from build123d import *

# Parameters (mm, degrees)
SKETCH_1_W          = 204
SKETCH_1_H          = 52
EXTRUDE_1_DEPTH     = 6
CUT_EXTRUDE_1_REACH = 107.432
SKETCH_2_R          = 1.6
SKETCH_2_R_2        = 4.5
FILLET_3_R          = 20


with BuildPart() as part:
    # 草图1 → 凸台-拉伸1 (new body)
    with BuildSketch(Plane.XY):
        Rectangle(SKETCH_1_W, SKETCH_1_H)
    extrude(amount=EXTRUDE_1_DEPTH)

    # 草图2 → 切除-拉伸1 (cut, up to next)
    with BuildSketch(Plane.XY.offset(6), mode=Mode.PRIVATE) as cut_extrude_1_sk1:
        with Locations((-91.5, 15.5)):
            Circle(SKETCH_2_R)
    cut_extrude_1_tool1 = extrude(cut_extrude_1_sk1.sketch, amount=-CUT_EXTRUDE_1_REACH, mode=Mode.PRIVATE) & part.part
    # 草图2 → 切除-拉伸1 (cut, up to next)
    with BuildSketch(Plane.XY.offset(6), mode=Mode.PRIVATE) as cut_extrude_1_sk2:
        with Locations((-60.5, 15.5)):
            Circle(SKETCH_2_R)
    cut_extrude_1_tool2 = extrude(cut_extrude_1_sk2.sketch, amount=-CUT_EXTRUDE_1_REACH, mode=Mode.PRIVATE) & part.part
    # 草图2 → 切除-拉伸1 (cut, up to next)
    with BuildSketch(Plane.XY.offset(6), mode=Mode.PRIVATE) as cut_extrude_1_sk3:
        with Locations((-91.5, -15.5)):
            Circle(SKETCH_2_R)
    cut_extrude_1_tool3 = extrude(cut_extrude_1_sk3.sketch, amount=-CUT_EXTRUDE_1_REACH, mode=Mode.PRIVATE) & part.part
    # 草图2 → 切除-拉伸1 (cut, up to next)
    with BuildSketch(Plane.XY.offset(6), mode=Mode.PRIVATE) as cut_extrude_1_sk4:
        with Locations((-60.5, -15.5)):
            Circle(SKETCH_2_R)
    cut_extrude_1_tool4 = extrude(cut_extrude_1_sk4.sketch, amount=-CUT_EXTRUDE_1_REACH, mode=Mode.PRIVATE) & part.part
    # 草图2 → 切除-拉伸1 (cut, up to next)
    with BuildSketch(Plane.XY.offset(6), mode=Mode.PRIVATE) as cut_extrude_1_sk5:
        with Locations((60.5, 15.5)):
            Circle(SKETCH_2_R)
    cut_extrude_1_tool5 = extrude(cut_extrude_1_sk5.sketch, amount=-CUT_EXTRUDE_1_REACH, mode=Mode.PRIVATE) & part.part
    # 草图2 → 切除-拉伸1 (cut, up to next)
    with BuildSketch(Plane.XY.offset(6), mode=Mode.PRIVATE) as cut_extrude_1_sk6:
        with Locations((91.5, 15.5)):
            Circle(SKETCH_2_R)
    cut_extrude_1_tool6 = extrude(cut_extrude_1_sk6.sketch, amount=-CUT_EXTRUDE_1_REACH, mode=Mode.PRIVATE) & part.part
    # 草图2 → 切除-拉伸1 (cut, up to next)
    with BuildSketch(Plane.XY.offset(6), mode=Mode.PRIVATE) as cut_extrude_1_sk7:
        with Locations((91.5, -15.5)):
            Circle(SKETCH_2_R)
    cut_extrude_1_tool7 = extrude(cut_extrude_1_sk7.sketch, amount=-CUT_EXTRUDE_1_REACH, mode=Mode.PRIVATE) & part.part
    # 草图2 → 切除-拉伸1 (cut, up to next)
    with BuildSketch(Plane.XY.offset(6), mode=Mode.PRIVATE) as cut_extrude_1_sk8:
        with Locations((60.5, -15.5)):
            Circle(SKETCH_2_R)
    cut_extrude_1_tool8 = extrude(cut_extrude_1_sk8.sketch, amount=-CUT_EXTRUDE_1_REACH, mode=Mode.PRIVATE) & part.part
    # 草图2 → 切除-拉伸1 (cut, up to next)
    with BuildSketch(Plane.XY.offset(6), mode=Mode.PRIVATE) as cut_extrude_1_sk9:
        with Locations((-76, 0)):
            Circle(SKETCH_2_R_2)
    cut_extrude_1_tool9 = extrude(cut_extrude_1_sk9.sketch, amount=-CUT_EXTRUDE_1_REACH, mode=Mode.PRIVATE) & part.part
    # 草图2 → 切除-拉伸1 (cut, up to next)
    with BuildSketch(Plane.XY.offset(6), mode=Mode.PRIVATE) as cut_extrude_1_sk10:
        with Locations((76, 0)):
            Circle(SKETCH_2_R_2)
    cut_extrude_1_tool10 = extrude(cut_extrude_1_sk10.sketch, amount=-CUT_EXTRUDE_1_REACH, mode=Mode.PRIVATE) & part.part
    # 草图2 → 切除-拉伸1 (cut, up to next)
    with BuildSketch(Plane.XY.offset(6), mode=Mode.PRIVATE) as cut_extrude_1_sk11:
        with BuildLine():
            Line((-46.5, 17.1), (-41.5, 17.1))
            ThreePointArc((-41.5, 17.1), (-39.9, 15.5), (-41.5, 13.9))
            Line((-41.5, 13.9), (-46.5, 13.9))
            ThreePointArc((-46.5, 13.9), (-48.1, 15.5), (-46.5, 17.1))
        make_face()
    cut_extrude_1_tool11 = extrude(cut_extrude_1_sk11.sketch, amount=-CUT_EXTRUDE_1_REACH, mode=Mode.PRIVATE) & part.part
    # 草图2 → 切除-拉伸1 (cut, up to next)
    with BuildSketch(Plane.XY.offset(6), mode=Mode.PRIVATE) as cut_extrude_1_sk12:
        with BuildLine():
            Line((-15.5, 17.1), (-10.5, 17.1))
            ThreePointArc((-10.5, 17.1), (-8.9, 15.5), (-10.5, 13.9))
            Line((-10.5, 13.9), (-15.5, 13.9))
            ThreePointArc((-15.5, 13.9), (-17.1, 15.5), (-15.5, 17.1))
        make_face()
    cut_extrude_1_tool12 = extrude(cut_extrude_1_sk12.sketch, amount=-CUT_EXTRUDE_1_REACH, mode=Mode.PRIVATE) & part.part
    # 草图2 → 切除-拉伸1 (cut, up to next)
    with BuildSketch(Plane.XY.offset(6), mode=Mode.PRIVATE) as cut_extrude_1_sk13:
        with BuildLine():
            Line((-46.5, -13.9), (-41.5, -13.9))
            ThreePointArc((-41.5, -13.9), (-39.9, -15.5), (-41.5, -17.1))
            Line((-41.5, -17.1), (-46.5, -17.1))
            ThreePointArc((-46.5, -17.1), (-48.1, -15.5), (-46.5, -13.9))
        make_face()
    cut_extrude_1_tool13 = extrude(cut_extrude_1_sk13.sketch, amount=-CUT_EXTRUDE_1_REACH, mode=Mode.PRIVATE) & part.part
    # 草图2 → 切除-拉伸1 (cut, up to next)
    with BuildSketch(Plane.XY.offset(6), mode=Mode.PRIVATE) as cut_extrude_1_sk14:
        with BuildLine():
            Line((-15.5, -13.9), (-10.5, -13.9))
            ThreePointArc((-10.5, -13.9), (-8.9, -15.5), (-10.5, -17.1))
            Line((-10.5, -17.1), (-15.5, -17.1))
            ThreePointArc((-15.5, -17.1), (-17.1, -15.5), (-15.5, -13.9))
        make_face()
    cut_extrude_1_tool14 = extrude(cut_extrude_1_sk14.sketch, amount=-CUT_EXTRUDE_1_REACH, mode=Mode.PRIVATE) & part.part
    # 草图2 → 切除-拉伸1 (cut, up to next)
    with BuildSketch(Plane.XY.offset(6), mode=Mode.PRIVATE) as cut_extrude_1_sk15:
        with BuildLine():
            Line((10.5, 17.1), (15.5, 17.1))
            ThreePointArc((15.5, 17.1), (17.1, 15.5), (15.5, 13.9))
            Line((15.5, 13.9), (10.5, 13.9))
            ThreePointArc((10.5, 13.9), (8.9, 15.5), (10.5, 17.1))
        make_face()
    cut_extrude_1_tool15 = extrude(cut_extrude_1_sk15.sketch, amount=-CUT_EXTRUDE_1_REACH, mode=Mode.PRIVATE) & part.part
    # 草图2 → 切除-拉伸1 (cut, up to next)
    with BuildSketch(Plane.XY.offset(6), mode=Mode.PRIVATE) as cut_extrude_1_sk16:
        with BuildLine():
            Line((41.5, 17.1), (46.5, 17.1))
            ThreePointArc((46.5, 17.1), (48.1, 15.5), (46.5, 13.9))
            Line((46.5, 13.9), (41.5, 13.9))
            ThreePointArc((41.5, 13.9), (39.9, 15.5), (41.5, 17.1))
        make_face()
    cut_extrude_1_tool16 = extrude(cut_extrude_1_sk16.sketch, amount=-CUT_EXTRUDE_1_REACH, mode=Mode.PRIVATE) & part.part
    # 草图2 → 切除-拉伸1 (cut, up to next)
    with BuildSketch(Plane.XY.offset(6), mode=Mode.PRIVATE) as cut_extrude_1_sk17:
        with BuildLine():
            Line((10.5, -13.9), (15.5, -13.9))
            ThreePointArc((15.5, -13.9), (17.1, -15.5), (15.5, -17.1))
            Line((15.5, -17.1), (10.5, -17.1))
            ThreePointArc((10.5, -17.1), (8.9, -15.5), (10.5, -13.9))
        make_face()
    cut_extrude_1_tool17 = extrude(cut_extrude_1_sk17.sketch, amount=-CUT_EXTRUDE_1_REACH, mode=Mode.PRIVATE) & part.part
    # 草图2 → 切除-拉伸1 (cut, up to next)
    with BuildSketch(Plane.XY.offset(6), mode=Mode.PRIVATE) as cut_extrude_1_sk18:
        with BuildLine():
            Line((41.5, -13.9), (46.5, -13.9))
            ThreePointArc((46.5, -13.9), (48.1, -15.5), (46.5, -17.1))
            Line((46.5, -17.1), (41.5, -17.1))
            ThreePointArc((41.5, -17.1), (39.9, -15.5), (41.5, -13.9))
        make_face()
    cut_extrude_1_tool18 = extrude(cut_extrude_1_sk18.sketch, amount=-CUT_EXTRUDE_1_REACH, mode=Mode.PRIVATE) & part.part
    # 草图2 → 切除-拉伸1 (cut, up to next)
    with BuildSketch(Plane.XY.offset(6), mode=Mode.PRIVATE) as cut_extrude_1_sk19:
        with BuildLine():
            Line((-31, 2.5), (-26, 2.5))
            ThreePointArc((-26, 2.5), (-23.5, 0), (-26, -2.5))
            Line((-26, -2.5), (-31, -2.5))
            ThreePointArc((-31, -2.5), (-33.5, 0), (-31, 2.5))
        make_face()
    cut_extrude_1_tool19 = extrude(cut_extrude_1_sk19.sketch, amount=-CUT_EXTRUDE_1_REACH, mode=Mode.PRIVATE) & part.part
    # 草图2 → 切除-拉伸1 (cut, up to next)
    with BuildSketch(Plane.XY.offset(6), mode=Mode.PRIVATE) as cut_extrude_1_sk20:
        with BuildLine():
            Line((26, 2.5), (31, 2.5))
            ThreePointArc((31, 2.5), (33.5, 0), (31, -2.5))
            Line((31, -2.5), (26, -2.5))
            ThreePointArc((26, -2.5), (23.5, 0), (26, 2.5))
        make_face()
    cut_extrude_1_tool20 = extrude(cut_extrude_1_sk20.sketch, amount=-CUT_EXTRUDE_1_REACH, mode=Mode.PRIVATE) & part.part
    add(cut_extrude_1_tool1.solids().sort_by_distance((-91.5, 15.5, 6))[0], mode=Mode.SUBTRACT)
    add(cut_extrude_1_tool2.solids().sort_by_distance((-60.5, 15.5, 6))[0], mode=Mode.SUBTRACT)
    add(cut_extrude_1_tool3.solids().sort_by_distance((-91.5, -15.5, 6))[0], mode=Mode.SUBTRACT)
    add(cut_extrude_1_tool4.solids().sort_by_distance((-60.5, -15.5, 6))[0], mode=Mode.SUBTRACT)
    add(cut_extrude_1_tool5.solids().sort_by_distance((60.5, 15.5, 6))[0], mode=Mode.SUBTRACT)
    add(cut_extrude_1_tool6.solids().sort_by_distance((91.5, 15.5, 6))[0], mode=Mode.SUBTRACT)
    add(cut_extrude_1_tool7.solids().sort_by_distance((91.5, -15.5, 6))[0], mode=Mode.SUBTRACT)
    add(cut_extrude_1_tool8.solids().sort_by_distance((60.5, -15.5, 6))[0], mode=Mode.SUBTRACT)
    add(cut_extrude_1_tool9.solids().sort_by_distance((-76, 0, 6))[0], mode=Mode.SUBTRACT)
    add(cut_extrude_1_tool10.solids().sort_by_distance((76, 0, 6))[0], mode=Mode.SUBTRACT)
    add(cut_extrude_1_tool11.solids().sort_by_distance((-44, 15.5, 6))[0], mode=Mode.SUBTRACT)
    add(cut_extrude_1_tool12.solids().sort_by_distance((-13, 15.5, 6))[0], mode=Mode.SUBTRACT)
    add(cut_extrude_1_tool13.solids().sort_by_distance((-44, -15.5, 6))[0], mode=Mode.SUBTRACT)
    add(cut_extrude_1_tool14.solids().sort_by_distance((-13, -15.5, 6))[0], mode=Mode.SUBTRACT)
    add(cut_extrude_1_tool15.solids().sort_by_distance((13, 15.5, 6))[0], mode=Mode.SUBTRACT)
    add(cut_extrude_1_tool16.solids().sort_by_distance((44, 15.5, 6))[0], mode=Mode.SUBTRACT)
    add(cut_extrude_1_tool17.solids().sort_by_distance((13, -15.5, 6))[0], mode=Mode.SUBTRACT)
    add(cut_extrude_1_tool18.solids().sort_by_distance((44, -15.5, 6))[0], mode=Mode.SUBTRACT)
    add(cut_extrude_1_tool19.solids().sort_by_distance((-28.5, 0, 6))[0], mode=Mode.SUBTRACT)
    add(cut_extrude_1_tool20.solids().sort_by_distance((28.5, 0, 6))[0], mode=Mode.SUBTRACT)

    # 圆角3
    fillet_3_edges = [part.edges().sort_by_distance(p)[0] for p in [
        (-102, 26, 3),
        (102, 26, 3),
        (102, -26, 3),
        (-102, -26, 3),
    ]]
    fillet(fillet_3_edges, radius=FILLET_3_R)


solid = part.part
CAD build for the part. Positions are in the model's coordinates, mm. Round coordinates to 2 decimals unless told otherwise and drop trailing zeros. Loops run counter-clockwise (first coordinate to the right, second up) from the corner with the lowest first, then second, coordinate; pieces in that order, holes last. Notation, with made-up numbers: M 0.5,62.25 L 45.5,62.25 A13 cw 45.5,66.25 Z; hole C 38,24.5 d1. An arc over 180 degrees is marked long. One line per question, with ' | ' between items. Start each with the question number.
Item 1: Cut at A-A, the plane x = -77. Write the cut outline in (y, z), plus the area to 3 significant figures.
Item 2: Wall check: line 1 (Y direction, x = 15, z = 4.85); line 2 (Y direction, x = 76, z = 2.9); line 3 (Y direction, x = -72, z = 5.05). Give the ranges that are in metal, low to high.
Item 3: Cut at C-C, the plane y = 22. Write the cut outline in (x, z).
Item 4: Cut at B-B, the plane z = 1.8. State how many separate pieces and enclosed holes the cut face has, plus the area to 3 significant figures.
Item 5: Pin check, flat tips, straight feed: pin 1 Ø3 at (y, z) = (-12, 5) entering from -X; pin 2 Ø1 at (y, z) = (-12.5, 4.5) entering from +X. Stop position of each tip, or through.
Responses:
1) outline: M -26,0 L -4.39,0 L -4.39,6 L -26,6 Z; M 4.39,0 L 26,0 L 26,6 L 4.39,6 Z | area: 259 mm²
2) line 1: y = -26 to -17.1, -13.9 to 13.9, 17.1 to 26 | line 2: y = -26 to -4.5, 4.5 to 26 | line 3: y = -26 to -2.06, 2.06 to 26
3) outline: M -94,0 L 94,0 L 94,6 L -94,6 Z
4) separate pieces: 1 | enclosed holes: 20 | area: 9,790 mm²
5) pin 1: stops at x = -101.49 | pin 2: stops at x = 101.08
